```python
from build123d import *

# Parameters (mm, degrees)
SKETCH1_W                = 97
SKETCH1_H                = 49.5
SKETCH1_R                = 1.5
BOSS_EXTRUDE1_DEPTH      = 1.6
SKETCH2_W                = 26.8
SKETCH2_H                = 6.5
SKETCH2_W_2              = 16.5
SKETCH2_W_3              = 21
SKETCH2_H_2              = 9.5
BOSS_EXTRUDE2_DEPTH      = 9.5
SKETCH2_3_W              = 53
SKETCH2_3_H              = 21
SKETCH2_3_W_2            = 16
SKETCH2_3_H_2            = 9
BOSS_EXTRUDE3_DEPTH      = 4.7
SKETCH2_4_W              = 8
SKETCH2_4_H              = 6
BOSS_EXTRUDE4_DEPTH      = 17
SKETCH3_R                = 1
BOSS_EXTRUDE5_DEPTH      = 1
BOSS_EXTRUDE6_DEPTH      = 0.1
BOSS_EXTRUDE6_DEPTH_BACK = 8


with BuildPart() as part:
    # Sketch1 → Boss-Extrude1 (new body)
    with BuildSketch(Plane(origin=(0, 0, 0), x_dir=(1, 0, 0), z_dir=(0, 1, 0))):
        Rectangle(SKETCH1_W, SKETCH1_H)
        with Locations(Location((-43.18, 17.78, 0), (0, 0, 270))):
            Circle(SKETCH1_R, mode=Mode.SUBTRACT)
        with Locations(Location((-43.18, -17.78, 0), (0, 0, 270))):
            Circle(SKETCH1_R, mode=Mode.SUBTRACT)
        with Locations(Location((43.18, 17.78, 0), (0, 0, 270))):
            Circle(SKETCH1_R, mode=Mode.SUBTRACT)
        with Locations(Location((43.18, -17.78, 0), (0, 0, 270))):
            Circle(SKETCH1_R, mode=Mode.SUBTRACT)
    extrude(amount=BOSS_EXTRUDE1_DEPTH)

    # Sketch2 → Boss-Extrude2 (add)
    with BuildSketch(Plane(origin=(0, 1.6, 0), x_dir=(1, 0, 0), z_dir=(0, 1, 0))):
        with Locations((11.6, 20)):
            Rectangle(SKETCH2_W, SKETCH2_H)
        with Locations((-13.75, 20)):
            Rectangle(SKETCH2_W_2, SKETCH2_H)
        with Locations((-20.5, -17)):
            Rectangle(SKETCH2_W_3, SKETCH2_H_2)
    extrude(amount=BOSS_EXTRUDE2_DEPTH)

    # Sketch2_3 → Boss-Extrude3 (add)
    with BuildSketch(Plane(origin=(0, 1.6, 0), x_dir=(1, 0, 0), z_dir=(0, 1, 0))):
        with Locations((-20.5, 2.75)):
            Rectangle(SKETCH2_3_W, SKETCH2_3_H)
        with Locations((14.5, -1.75)):
            Rectangle(SKETCH2_3_W_2, SKETCH2_3_H_2)
        with Locations((14.5, 7.25)):
            Rectangle(SKETCH2_3_W_2, SKETCH2_3_H_2)
    extrude(amount=BOSS_EXTRUDE3_DEPTH)

    # Sketch2_4 → Boss-Extrude4 (add)
    with BuildSketch(Plane(origin=(0, 1.6, 0), x_dir=(1, 0, 0), z_dir=(0, 1, 0))):
        with Locations((13.2, -14.25)):
            Rectangle(SKETCH2_4_W, SKETCH2_4_H)
    extrude(amount=BOSS_EXTRUDE4_DEPTH)

    # Sketch3 → Boss-Extrude5 (add)
    with BuildSketch(Plane(origin=(0, 6.3, 0), x_dir=(1, 0, 0), z_dir=(0, 1, 0))):
        with Locations(Location((-5, 7.25, 0), (0, 0, 270))):
            Circle(SKETCH3_R)
    extrude(amount=BOSS_EXTRUDE5_DEPTH)

    # Sketch4 → Boss-Extrude6 (add, two sides: drawn at the far end of the back side and taken through both)
    with BuildSketch(Plane.ZY.offset(47).offset(-BOSS_EXTRUDE6_DEPTH_BACK)):
        with BuildLine():
            Line((-5.65, 10.3), (0.15, 10.3))
            ThreePointArc((0.15, 10.3), (2.15, 8.3), (0.15, 6.3))
            Line((0.15, 6.3), (-5.65, 6.3))
            ThreePointArc((-5.65, 6.3), (-7.65, 8.3), (-5.65, 10.3))
        make_face()
    extrude(amount=BOSS_EXTRUDE6_DEPTH + BOSS_EXTRUDE6_DEPTH_BACK)


solid = part.part
```
Design review of the part built by this model. Coordinates are the model's own, in mm. A direction names the side the tool comes from. Give positions to 0.01 mm unless a question says otherwise; leave off trailing zeros. Write each loop counter-clockwise with the first axis right and the second up, starting at its lowest first coordinate (ties: lowest second). Pieces come first, ordered by that corner, then holes.
(1) Add section D-D (x = 24). Give the boundary of the cut face in (y, z), and give its area (3 significant figures).
Checked values:
outline: (0, -24.75) - (1.6, -24.75) - (1.6, -23.25) - (11.1, -23.25) - (11.1, -16.75) - (1.6, -16.75) - (1.6, 24.75) - (0, 24.75) - close
area: 141 mm2
(2) Clearance check with flat-ended pins moving along their axes: pin 1 Ø10 at (x, z) = (34, 9.5) entering from -Y; pin 2 Ø3 at (x, z) = (-43, -3) entering from +Y; pin 3 Ø2 at (y, z) = (4.5, -20.5) entering from +X; pin 4 Ø3 at (y, z) = (8.5, 17) entering from +X. State where each tip first meets the part, or that it passes through.
Checked values:
pin 1: stops at y = 0
pin 2: stops at y = 10.3
pin 3: stops at x = 25
pin 4: stops at x = 17.2
(3) Wall thickness on line 1 along X through (y, z) = (0.65, -17.78); line 2 along X through (y, z) = (6.75, 15.5); line 3 along Y through (x, z) = (-20, 5.5): over which ranges is each line inside the solid? List them lowest first.
Checked values:
line 1: x = -48.5 to -44.68, -41.68 to 41.68, 44.68 to 48.5
line 2: x = -31 to -10, 9.2 to 17.2
line 3: y = 0 to 6.3
(4) Add section A-A (x = 43.18). Give the boundary of the cut face in (y, z), and give its area (3 significant figures).
Checked values:
outline: (0, -24.75) - (1.6, -24.75) - (1.6, -19.28) - (0, -19.28) - close; (0, -16.28) - (1.6, -16.28) - (1.6, 16.28) - (0, 16.28) - close; (0, 19.28) - (1.6, 19.28) - (1.6, 24.75) - (0, 24.75) - close
area: 69.6 mm2
(5) Add section C-C (z = -17.78). Give the boundary of the cut face in (x, y).
Checked values:
outline: (-48.5, 0) - (-44.68, 0) - (-44.68, 1.6) - (-48.5, 1.6) - close; (-41.68, 0) - (41.68, 0) - (41.68, 1.6) - (25, 1.6) - (25, 11.1) - (-1.8, 11.1) - (-1.8, 1.6) - (-5.5, 1.6) - (-5.5, 11.1) - (-22, 11.1) - (-22, 1.6) - (-41.68, 1.6) - close; (44.68, 0) - (48.5, 0) - (48.5, 1.6) - (44.68, 1.6) - close
(6) Mouldability with a two-part tool opening along X and no side actions: class faces 1 (the face through (-42.7, 0.8, 19.2)), 2 (the face through (11, 6, -16.75)), 3 (the face through (17.2, 10, 14)) as +X half, -X half, draft (parallel to the pull), parting line (faces both ways), or undercut.
Checked values:
face 1: undercut
face 2: draft
face 3: +X half
(7) Add section B-B (y = 4.75). Give the boundary of the cut face in (x, z).
Checked values:
outline: (-47, -13.25) - (6, -13.25) - (6, 7.75) - (-47, 7.75) - close; (-31, 12.25) - (-10, 12.25) - (-10, 21.75) - (-31, 21.75) - close; (-22, -23.25) - (-5.5, -23.25) - (-5.5, -16.75) - (-22, -16.75) - close; (-1.8, -23.25) - (25, -23.25) - (25, -16.75) - (-1.8, -16.75) - close; (6.5, -11.75) - (22.5, -11.75) - (22.5, 6.25) - (6.5, 6.25) - close; (9.2, 11.25) - (17.2, 11.25) - (17.2, 17.25) - (9.2, 17.25) - close
(8) Tool access review of faces 4 (the face through (9.2, 10, 14)), 5 (the face through (-21, 6, 21.75)), 6 (the face through (13, 10, 11.25)), 7 (the face through (14, 4, 6.25)), 8 (the face through (-5, 7.3, -7)): name each direction out of +Z, -Z, +X, -X, +Y, -Y from which nothing blocks a thin tool from reaching the whole face with its end or side.
Checked values:
face 4: +Z, +Y
face 5: +Z, +X, -X, +Y
face 6: +X, -X, +Y
face 7: +X, +Y
face 8: +Z, +X, +Y
